Check sheet for the modelled part. Datum: model origin and axes. Units: mm. Give positions to 0.01 mm unless a question says otherwise; leave off trailing zeros. Loops run counter-clockwise (first coordinate to the right, second up) from the corner with the lowest first, then second, coordinate; pieces in that order, holes last. Notation, with made-up numbers: (38, 78.25) - (85, 78.25) arc R21 ccw to (85, 98.25) - close; hole circle Ø3 at (-25, 46.25). An arc over 180 degrees is marked (long way). Answer in a Markdown table with one row per item. Add a question column.
(1) Thickness scan on L1, parallel to Z at x = 0, y = -2.5 (3 decimals); L2, parallel to Z at x = 34, y = -7.5; L3, parallel to Z at x = -41, y = -3. Record the ranges inside material, lowest first.
(2) Sectioned sample at B-B on x = 19. Enter the section's corners in (y, z) (3 decimals), then the cut area to 3 significant figures.
(3) Draft check along X on faces 1 (the face through (47.88, -6.08, 7.46)), 2 (the face through (-1, -6, 160)), 3 (the face through (-60, -6, 79)). Enter one of: released by +X, released by -X, zero draft, split by the parting line, or undercut.
(4) Sectioned sample at A-A on x = 5.83. Enter the section's corners in (y, z) (3 decimals).
from build123d import *

# Parameters (mm, degrees)
SKETCH_W      = 120
SKETCH_H      = 160
PAD_DEPTH     = 12
SKETCH001_R   = 2.25
SKETCH001_R_2 = 3
POCKET_DEPTH  = 12.001


with BuildPart() as part:
    # Sketch → Pad (new body)
    with BuildSketch(Plane.XZ):
        with Locations((0, 80)):
            Rectangle(SKETCH_W, SKETCH_H)
    extrude(amount=PAD_DEPTH)

    # Sketch001 → Pocket (cut, through all)
    with BuildSketch(Plane.XZ.offset(12)):
        with Locations((-45.83, 37.375)):
            Circle(SKETCH001_R)
        with Locations((-34.17, 8.325)):
            Circle(SKETCH001_R)
        with Locations((34.144, 37.375)):
            Circle(SKETCH001_R)
        with Locations((45.804, 8.325)):
            Circle(SKETCH001_R)
        with Locations((-5.83, 151.675)):
            Circle(SKETCH001_R)
        with Locations((5.83, 122.625)):
            Circle(SKETCH001_R)
        with Locations((-49.725, 72.97)):
            Circle(SKETCH001_R)
        with Locations((49.725, 72.97)):
            Circle(SKETCH001_R)
        with Locations((0, 108.025)):
            Circle(SKETCH001_R)
        with Locations((-19, 52.375)):
            Circle(SKETCH001_R_2)
        with Locations((19, 52.375)):
            Circle(SKETCH001_R_2)
        with Locations((0, 6)):
            Circle(SKETCH001_R)
        with Locations((-41, 152.5)):
            Circle(SKETCH001_R)
        with Locations((41, 152.5)):
            Circle(SKETCH001_R)
        with Locations((-42.5, 110)):
            Circle(SKETCH001_R)
        with Locations((42.5, 110)):
            Circle(SKETCH001_R)
    extrude(amount=-POCKET_DEPTH, mode=Mode.SUBTRACT)


solid = part.part
Reply:
| question | item | result |
|---|---|---|
| 1 | L1 | 0 to 3.75, 8.25 to 105.775, 110.275 to 160 |
| 1 | L2 | 0 to 35.13, 39.62 to 160 |
| 1 | L3 | 0 to 108.32, 111.68 to 150.25, 154.75 to 160 |
| 2 | outline | (-12, 0) - (0, 0) - (0, 49.375) - (-12, 49.375) - close; (-12, 55.375) - (0, 55.375) - (0, 160) - (-12, 160) - close |
| 2 | area | 1,850 mm^2 |
| 3 | face 1 | undercut |
| 3 | face 2 | zero draft |
| 3 | face 3 | released by -X |
| 4 | outline | (-12, 0) - (0, 0) - (0, 120.375) - (-12, 120.375) - close; (-12, 124.875) - (0, 124.875) - (0, 160) - (-12, 160) - close |
